from build123d import *

# Parameters (mm, degrees)
F0_R     = 11.125
F1_DEPTH = 5


with BuildPart() as f1:
    # F0 (on Top) → F1 (new body)
    with BuildSketch(Plane.XY):
        Polygon((25.034333, -2.465667), (27.5, 0), (25.034333, 2.465667), (26.971595, 5.364984), (24.072278, 7.302246), (25.406687, 10.523794), (22.185138, 11.858204), (22.865414, 15.278181), (19.445436, 15.958457), (19.445436, 19.445436), (15.958457, 19.445436), (15.278181, 22.865414), (11.858204, 22.185138), (10.523794, 25.406687), (7.302246, 24.072278), (5.364984, 26.971595), (2.465667, 25.034333), (0, 27.5), (-2.465667, 25.034333), (-5.364984, 26.971595), (-7.302246, 24.072278), (-10.523794, 25.406687), (-11.858204, 22.185138), (-15.278181, 22.865414), (-15.958457, 19.445436), (-19.445436, 19.445436), (-19.445436, 15.958457), (-22.865414, 15.278181), (-22.185138, 11.858204), (-25.406687, 10.523794), (-24.072278, 7.302246), (-26.971595, 5.364984), (-25.034333, 2.465667), (-27.5, 0), (-25.034333, -2.465667), (-26.971595, -5.364984), (-24.072278, -7.302246), (-25.406687, -10.523794), (-22.185138, -11.858204), (-22.865414, -15.278181), (-19.445436, -15.958457), (-19.445436, -19.445436), (-15.958457, -19.445436), (-15.278181, -22.865414), (-11.858204, -22.185138), (-10.523794, -25.406687), (-7.302246, -24.072278), (-5.364984, -26.971595), (-2.465667, -25.034333), (0, -27.5), (2.465667, -25.034333), (5.364984, -26.971595), (7.302246, -24.072278), (10.523794, -25.406687), (11.858204, -22.185138), (15.278181, -22.865414), (15.958457, -19.445436), (19.445436, -19.445436), (19.445436, -15.958457), (22.865414, -15.278181), (22.185138, -11.858204), (25.406687, -10.523794), (24.072278, -7.302246), (26.971595, -5.364984), align=None)
        Circle(F0_R, mode=Mode.SUBTRACT)
    extrude(amount=F1_DEPTH)


solid = f1.part
Here's how the part is built. I have some questions about the finished solid (model axes, mm). A direction names the side the tool comes from. Round coordinates to 2 decimals unless told otherwise and drop trailing zeros. Loops run counter-clockwise (first coordinate to the right, second up) from the corner with the lowest first, then second, coordinate; pieces in that order, holes last. Notation, with made-up numbers: (23.5, 89.25) -> (81.5, 89.25) arc R33 ccw to (81.5, 126.25) -> close; hole circle Ø8 at (36.25, 79). An arc over 180 degrees is marked (long way). Write each question's results on one line, items separated by ' | '.
(1) We'd pull the mould along X, two halves only. Please class faces 1 (the face through (23.82, 11.18, 2.46)), 2 (the face through (-26.2, 1.3, 2.5)), 3 (the face through (-1.2, 26.3, 2.5)): released by +X, released by -X, zero draft, split by the parting line, or undercut.
Worked answers:
face 1: released by +X | face 2: released by -X | face 3: undercut
(2) If we section it at B-B, the plane y = 17.5: List the corners of the cut face in (x, z) for me, then the cut area to 3 significant figures.
Worked answers:
outline: (-19.45, 0) -> (19.45, 0) -> (19.45, 5) -> (-19.45, 5) -> close | area: 194 mm2
(3) For faces 4 (the face through (24.73, 8.89, 2.46)), 5 (the face through (8.94, 24.75, 2.46)), 6 (the face through (21.131, -15.623, 2.465)), 7 (the face through (-11.2, -23.77, 2.46)), 8 (the face through (-26.02, 3.94, 2.46)), which set-ups out of +Z, -Z, +X, -X, +Y, -Y let a thin tool reach every point of the face, with its end or its side?
Worked answers:
face 4: +Z, -Z, +X | face 5: +Z, -Z, +Y | face 6: +Z, -Z, +X, -Y | face 7: +Z, -Z, -Y | face 8: +Z, -Z, -X
(4) For P1, Ø1, axis at y = 18, z = 3, coming from the +X side; P2, Ø3, axis at x = -6, z = 3.5, coming from the +Y side; P3, Ø1, axis at x = -1, z = 4.5, coming from the -Y side; P4, Ø1, axis at x = 8.5, y = -20.5, coming from the -Z side, each with a flat end and sliding along its axis, tell me the tip position at first contact or that it passes through.
Worked answers:
P1: x = 19.45 | P2: y = 26.97 | P3: y = -27 | P4: z = 0
(5) If we section it at A-A, the plane x = -6: List the corners of the cut face in (y, z) for me, then the cut area to 3 significant figures.
Worked answers:
outline: (-26.02, 0) -> (-9.37, 0) -> (-9.37, 5) -> (-26.02, 5) -> close; (9.37, 0) -> (26.02, 0) -> (26.02, 5) -> (9.37, 5) -> close | area: 167 mm2
(6) If I drill on L1, parallel to X at y = -19, z = 3.45; L2, parallel to Y at x = -0.5, z = 4.4, over which ranges is the centre line in solid material (lowest first)?
Worked answers:
L1: -19.45 to 19.45 | L2: -27 to -11.11, 11.11 to 27
